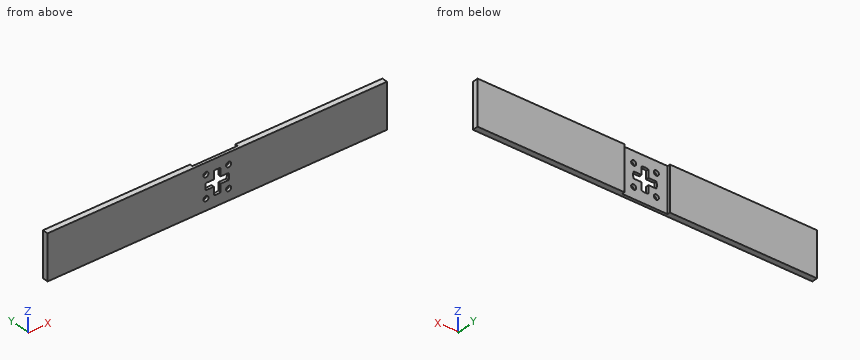
from build123d import *

# Parameters (mm, degrees)
SKETCH1_W           = 300
SKETCH1_H           = 40
SKETCH1_R           = 2.25
BOSS_EXTRUDE1_DEPTH = 2.5
SKETCH2_W           = 40
SKETCH2_H           = 2.5
CUT_EXTRUDE1_DEPTH  = 156.261875552


with BuildPart() as part:
    # Sketch1 → Boss-Extrude1 (new, symmetric)
    with BuildSketch(Plane(origin=(0, 0, 0), x_dir=(1, 0, 0), z_dir=(0, 1, 0))):
        Rectangle(SKETCH1_W, SKETCH1_H)
        with Locations(Location((10, -10, 0), (0, 0, 270))):
            Circle(SKETCH1_R, mode=Mode.SUBTRACT)
        with Locations(Location((10, 10, 0), (0, 0, 90))):
            Circle(SKETCH1_R, mode=Mode.SUBTRACT)
        with Locations(Location((-10, -10, 0), (0, 0, 90))):
            Circle(SKETCH1_R, mode=Mode.SUBTRACT)
        with Locations(Location((-10, 10, 0), (0, 0, 270))):
            Circle(SKETCH1_R, mode=Mode.SUBTRACT)
        with BuildLine():
            Line((-3, -3), (-3, -10.062305899))
            ThreePointArc((-3, -10.062305899), (0, -10.5), (3, -10.062305899))
            Line((3, -10.062305899), (3, -3))
            Line((3, -3), (10.062305899, -3))
            ThreePointArc((10.062305899, -3), (10.5, 0), (10.062305899, 3))
            Line((10.062305899, 3), (3, 3))
            Line((3, 3), (3, 10.062305899))
            ThreePointArc((3, 10.062305899), (0, 10.5), (-3, 10.062305899))
            Line((-3, 10.062305899), (-3, 3))
            Line((-3, 3), (-10.062305899, 3))
            ThreePointArc((-10.062305899, 3), (-10.5, 0), (-10.062305899, -3))
            Line((-10.062305899, -3), (-3, -3))
        make_face(mode=Mode.SUBTRACT)
    extrude(amount=BOSS_EXTRUDE1_DEPTH, both=True)

    # Sketch2 → Cut-Extrude1 (cut, through all)
    with BuildSketch(Plane.XY.offset(20)):
        with Locations((0, 1.25)):
            Rectangle(SKETCH2_W, SKETCH2_H)
    extrude(amount=-CUT_EXTRUDE1_DEPTH, mode=Mode.SUBTRACT)


solid = part.part
For this review, take the finished solid that the model builds, in its own axes (mm). Round coordinates to 2 decimals unless told otherwise and drop trailing zeros. Loops run counter-clockwise (first coordinate to the right, second up) from the corner with the lowest first, then second, coordinate; pieces in that order, holes last. Notation, with made-up numbers: (77.25, -35.5) - (81.25, -35.5) arc R4 cw to (81.25, -28.5) - close; hole circle Ø1 at (87, -8.5). An arc over 180 degrees is marked (long way). Use one line per item in the form item = value.
Item 1: Clearance check with a flat-ended pin moving along its axis: P1, Ø12, axis at x = 10, z = -5, coming from the +Y side. State where the tip first meets the part, or that it passes through.
Answers:
P1 = 0
Item 2: For line 1 (X direction, y = -1.9, z = -10); line 2 (Z direction, x = 10, y = -1.3); line 3 (X direction, y = -0.85, z = 0.5), list the stretches that pass through material, from the lowest coordinate up.
Answers:
line_1 = -150 to -12.25, -7.75 to -3, 3 to 7.75, 12.25 to 150
line_2 = -20 to -12.25, -7.75 to -3, 3 to 7.75, 12.25 to 20
line_3 = -150 to -10.49, 10.49 to 150
Item 3: Consider section C-C on z = -0.5. Write out the cut boundary in (x, y), then the cut area to 3 significant figures.
Answers:
outline = (-150, -2.5) - (-10.49, -2.5) - (-10.49, 0) - (-20, 0) - (-20, 2.5) - (-150, 2.5) - close; (10.49, -2.5) - (150, -2.5) - (150, 2.5) - (20, 2.5) - (20, 0) - (10.49, 0) - close
area = 1,350 mm^2
Item 4: Consider section B-B on z = 17.5. Write out the cut boundary in (x, y).
Answers:
outline = (-150, -2.5) - (150, -2.5) - (150, 2.5) - (20, 2.5) - (20, 0) - (-20, 0) - (-20, 2.5) - (-150, 2.5) - close
Item 5: Consider section A-A on y = 1.4. Write out the cut boundary in (x, z).
Answers:
outline = (-150, -20) - (-20, -20) - (-20, 20) - (-150, 20) - close; (20, -20) - (150, -20) - (150, 20) - (20, 20) - close
